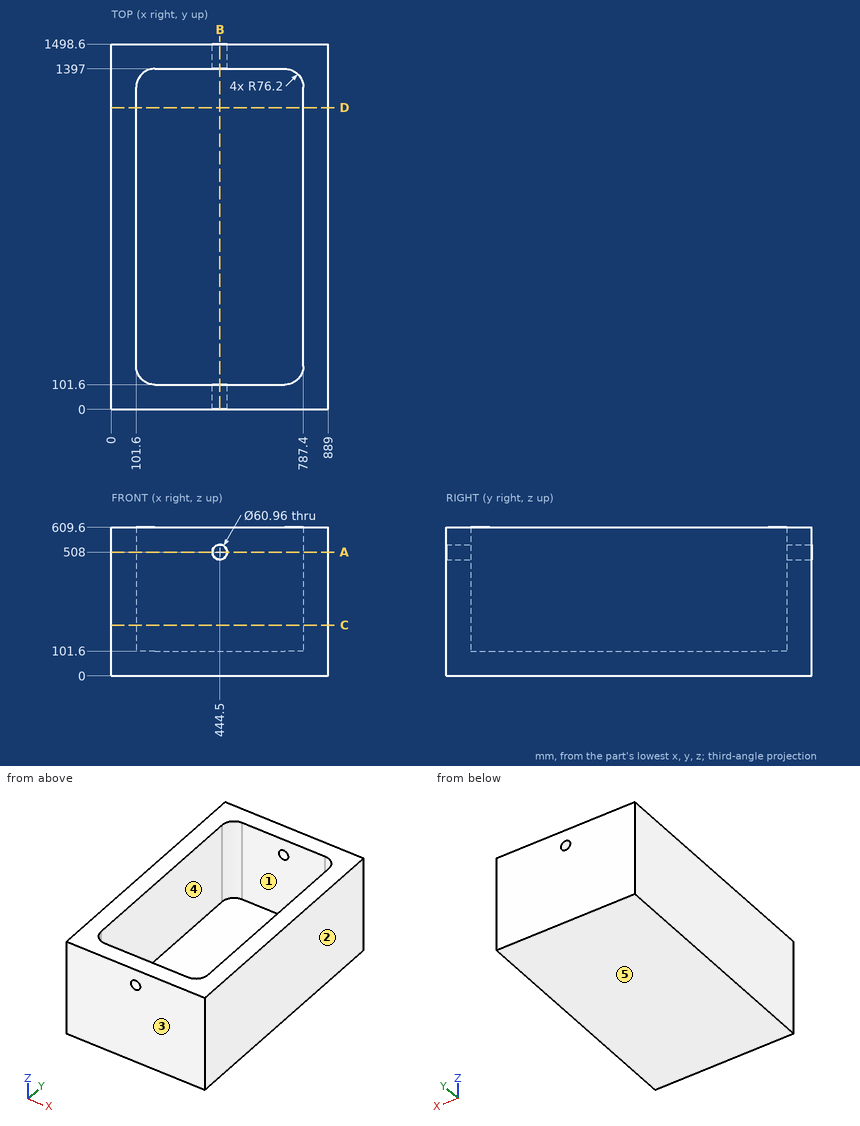
The figure shows three views and two pictorial views of one solid part (mm, origin at its lowest corner). Answer the questions. A direction names the side the tool comes from. Give positions to 0.01 mm unless a question says otherwise; leave off trailing zeros. Loops run counter-clockwise (first coordinate to the right, second up) from the corner with the lowest first, then second, coordinate; pieces in that order, holes last. Notation, with made-up numbers: M 66,31 L 117,31 A19 cw 117,41 Z; hole C -9,48 d10. An arc over 180 degrees is marked long. Write each question's results on one line, items separated by ' | '.
1. Given pin 1 (1 mm diameter, centred on x = 618.5, y = 981, fed in from -Z); pin 2 (1.5 mm diameter, centred on x = 466.5, y = 830, fed in from +Z), each flat-ended and moving along its own axis, determine where each tip first touches the part or whether it passes through.
Values:
pin 1: stops at z = 0 | pin 2: stops at z = 101.6
2. Section A-A on z = 508 is taken. Give the vertices of the cut face in (x, y), plus the area to 3 significant figures.
Values:
outline: M 0,0 L 414.02,0 L 414.02,101.6 L 177.8,101.6 A76.2 cw 101.6,177.8 L 101.6,1320.8 A76.2 cw 177.8,1397 L 414.02,1397 L 414.02,1498.6 L 0,1498.6 Z; M 474.98,0 L 889,0 L 889,1498.6 L 474.98,1498.6 L 474.98,1397 L 711.2,1397 A76.2 cw 787.4,1320.8 L 787.4,177.8 A76.2 cw 711.2,101.6 L 474.98,101.6 Z | area: 436,000 mm^2
3. Straight lines are drawn through the part: line 1 (X direction, y = 1460.5, z = 508); line 2 (X direction, y = 877, z = 396); line 3 (Z direction, x = 444.5, y = 69). For each, find the intervals that lie inside material, in ascending order. Write a range as [from, to].
Values:
line 1: x = [0, 414.02], [474.98, 889] | line 2: x = [0, 101.6], [787.4, 889] | line 3: z = [0, 477.52], [538.48, 609.6]
4. Section C-C on z = 208.5 is taken. Give the vertices of the cut face in (x, y).
Values:
outline: M 0,0 L 889,0 L 889,1498.6 L 0,1498.6 Z; hole M 101.6,177.8 A76.2 ccw 177.8,101.6 L 711.2,101.6 A76.2 ccw 787.4,177.8 L 787.4,1320.8 A76.2 ccw 711.2,1397 L 177.8,1397 A76.2 ccw 101.6,1320.8 Z
5. The mould has two halves that part along Y. Classify the marked faces 1, 2 and 3: pulls with the +Y half, pulls with the -Y half, needs draft (parallel to the pull), parting line crosses it, or undercut.
Values:
face 1: undercut | face 2: needs draft | face 3: pulls with the -Y half
6. A tool of negligible diameter and unlimited length cuts with its end or side. For the marked faces 4 and 5, from which of +Z, -Z, +X, -X, +Y, -Y can it reach the whole face along a straight path? Write none if from no direction.
Values:
face 4: +Z | face 5: -Z, +X, -X, +Y, -Y
7. Section B-B on x = 444.5 is taken. Give the vertices of the cut face in (y, z), plus the area to 3 significant figures.
Values:
outline: M 0,0 L 1498.6,0 L 1498.6,477.52 L 1397,477.52 L 1397,101.6 L 101.6,101.6 L 101.6,477.52 L 0,477.52 Z; M 0,538.48 L 101.6,538.48 L 101.6,609.6 L 0,609.6 Z; M 1397,538.48 L 1498.6,538.48 L 1498.6,609.6 L 1397,609.6 Z | area: 243,000 mm^2
8. Section D-D on y = 1237.5 is taken. Give the vertices of the cut face in (x, z).
Values:
outline: M 0,0 L 889,0 L 889,609.6 L 787.4,609.6 L 787.4,101.6 L 101.6,101.6 L 101.6,609.6 L 0,609.6 Z
